Model file for the job. Use its own axes, mm. A direction names the side the tool comes from. Round coordinates to 2 decimals unless told otherwise and drop trailing zeros. Loops run counter-clockwise (first coordinate to the right, second up) from the corner with the lowest first, then second, coordinate; pieces in that order, holes last.
from build123d import *

# Parameters (mm, degrees)
F1_DEPTH  = 50.8
F2_R      = 6.35
F3_W      = 38.1
F3_H      = 25.4
F4_DEPTH  = 38.1
F5_W      = 38.1
F5_H      = 25.4
F6_DEPTH  = 38.1
F7_W      = 101.6
F7_H      = 101.6
F8_DEPTH  = 76.2
F9_W      = 50.8
F9_H      = 25.4
F10_DEPTH = 152.401
F12_DEPTH = 76.2
F14_DEPTH = 76.2
F15_R     = 6.35


with BuildPart() as f1:
    # F0 (on Front) → F1 (new body, symmetric)
    with BuildSketch(Plane.XZ):
        Polygon((0, 25.4), (0, 0), (25.4, 0), (25.4, 25.4), (101.6, 25.4), (101.6, 0), (127, 0), (127, 25.4), (165.1, 25.4), (165.1, 50.8), (-38.1, 50.8), (-38.1, 25.4), align=None)
    extrude(amount=F1_DEPTH, both=True)

    # F2
    f2_edges = [f1.edges().sort_by_distance(p)[0] for p in [
        (-38.1, -50.8, 38.1),
        (165.1, -50.8, 38.1),
        (165.1, 50.8, 38.1),
        (-38.1, 50.8, 38.1),
    ]]
    fillet(f2_edges, radius=F2_R)

    # F3 (on face) → F4 (cut, through all)
    with BuildSketch(Plane.YZ.offset(165.1)):
        with Locations((0, 38.1)):
            Rectangle(F3_W, F3_H)
    extrude(amount=-F4_DEPTH, mode=Mode.SUBTRACT)

    # F5 (on face) → F6 (cut, through all)
    with BuildSketch(Plane(origin=(-38.1, 0, 0), x_dir=(0, -1, 0), z_dir=(-1, 0, 0))):
        with Locations((0, 38.1)):
            Rectangle(F5_W, F5_H)
    extrude(amount=-F6_DEPTH, mode=Mode.SUBTRACT)

    # F7 (on face) → F8 (join)
    with BuildSketch(Plane.XY.offset(50.8)):
        with Locations((63.5, 0)):
            Rectangle(F7_W, F7_H)
    extrude(amount=F8_DEPTH)

    # F9 (on face) → F10 (cut, through all)
    with BuildSketch(Plane.YZ.offset(114.3)):
        with Locations((-25.4, 88.9)):
            Rectangle(F9_W, F9_H)
    extrude(amount=-F10_DEPTH, mode=Mode.SUBTRACT)

    # F11 (on face) → F12 (cut, through all)
    with BuildSketch(Plane.XY.offset(127)):
        Polygon((63.5, -50.8), (12.7, 50.8), (12.7, -50.8), align=None)
    extrude(amount=-F12_DEPTH, mode=Mode.SUBTRACT)

    # F13 (on face) → F14 (cut, through all)
    with BuildSketch(Plane.XY.offset(127)):
        Polygon((114.3, 50.8), (63.5, -50.8), (114.3, -50.8), align=None)
    extrude(amount=-F14_DEPTH, mode=Mode.SUBTRACT)

    # F15
    f15_edges = [f1.edges().sort_by_distance(p)[0] for p in [
        (25.4, 0, 25.4),
        (101.6, 0, 25.4),
    ]]
    fillet(f15_edges, radius=F15_R)


solid = f1.part
Q1. Probe line 1 (Z direction, x = 54.5, y = -0.5); line 2 (Z direction, x = 65, y = 5); line 3 (Z direction, x = -22.5, y = -34). List the from-to ranges inside material, lowest first.
Q2. Slice it at B-B on x = -14. Give the cut face in (y, z), plus the area to 3 significant figures.
Q3. Slice it at D-D on z = 40.5. Give the cut face in (x, y).
Q4. Pull direction X, two halves, no side cores. Call faces 4 (the face through (163.29, -48.89, 38.28)), 5 (the face through (114, -1, 0)), 6 (the face through (-38.1, -32, 38)), 7 (the face through (25.4, -1, 9)): pulls with the +X half, pulls with the -X half, needs draft (parallel to the pull), parting line crosses it, or undercut.
Q5. Tool access for faces 1 (the face through (27.31, -0.71, 23.59)), 2 (the face through (64, 0, 89)), 3 (the face through (126, -12, 50.8)): list every direction of +Z, -Z, +X, -X, +Y, -Y with a clear straight run to the whole face (end or side of a thin tool).
Q6. Slice it at C-C on y = 7. Give the cut face in (x, z).
Q7. Slice it at A-A on y = -38. Give the cut face in (x, z).
Q8. Flat gauge pins, fed straight in: P1, Ø5, axis at x = 89.5, y = -28.5, coming from the +Z side; P2, Ø9.5, axis at y = 2.5, z = 8, coming from the +X side; P3, Ø9.5, axis at y = -5, z = 10.5, coming from the -X side. Where does each tip first touch, or does it go through?
Reply:
1. line 1: z = 25.4 to 76.2, 101.6 to 127
1. line 2: z = 25.4 to 127
1. line 3: z = 25.4 to 50.8
2. outline: (-50.8, 25.4) - (-19.05, 25.4) - (-19.05, 50.8) - (-50.8, 50.8) - close; (19.05, 25.4) - (50.8, 25.4) - (50.8, 50.8) - (19.05, 50.8) - close
2. area: 1,610 mm2
3. outline: (-38.1, -44.45) arc R6.35 ccw to (-31.75, -50.8) - (158.75, -50.8) arc R6.35 ccw to (165.1, -44.45) - (165.1, -19.05) - (127, -19.05) - (127, 19.05) - (165.1, 19.05) - (165.1, 44.45) arc R6.35 ccw to (158.75, 50.8) - (-31.75, 50.8) arc R6.35 ccw to (-38.1, 44.45) - (-38.1, 19.05) - (0, 19.05) - (0, -19.05) - (-38.1, -19.05) - close
4. face 4: pulls with the +X half
4. face 5: needs draft
4. face 6: pulls with the -X half
4. face 7: undercut
5. face 1: -Z, +Y, -Y
5. face 2: +X, -X, -Y
5. face 3: +Z, +X, -Y
6. outline: (0, 0) - (25.4, 0) - (25.4, 19.05) arc R6.35 cw to (31.75, 25.4) - (95.25, 25.4) arc R6.35 cw to (101.6, 19.05) - (101.6, 0) - (127, 0) - (127, 50.8) - (92.4, 50.8) - (92.4, 127) - (34.6, 127) - (34.6, 50.8) - (0, 50.8) - close
7. outline: (-38.1, 25.4) - (0, 25.4) - (0, 0) - (25.4, 0) - (25.4, 19.05) arc R6.35 cw to (31.75, 25.4) - (95.25, 25.4) arc R6.35 cw to (101.6, 19.05) - (101.6, 0) - (127, 0) - (127, 25.4) - (165.1, 25.4) - (165.1, 50.8) - (69.9, 50.8) - (69.9, 76.2) - (57.1, 76.2) - (57.1, 50.8) - (-38.1, 50.8) - close; (57.1, 101.6) - (69.9, 101.6) - (69.9, 127) - (57.1, 127) - close
8. P1: stops at z = 50.8
8. P2: stops at x = 127
8. P3: stops at x = 0
